```python
from build123d import *

# Parameters (mm, degrees)
EXTRUDE_1_DEPTH              = 5
SKETCH_2_R                   = 1.525
CUT_EXTRUDE_1_DEPTH          = 6
SKETCH_3_R                   = 48.25
EXTRUDE_2_DEPTH              = 5
SKETCH_4_R                   = 32
CUT_EXTRUDE_2_DEPTH          = 6
FILLET_1_R                   = 40
SKETCH_9_R                   = 7.5
CUT_EXTRUDE_7_DEPTH          = 6
SKETCH_15_R                  = 1.525
CUT_EXTRUDE_10_DEPTH         = 6
SKETCH_16_R                  = 1.525
SKETCH_16_R_2                = 3.525
CUT_EXTRUDE_11_DEPTH         = 6
SKETCH_17_R                  = 1.525
SKETCH_17_R_2                = 3.525
SKETCH_17_R_3                = 7.5
CUT_EXTRUDE_12_DEPTH         = 6
SKETCH_10_R                  = 1.775
CUT_EXTRUDE_13_DEPTH         = 6
SKETCH_19_R                  = 1.525
CUT_EXTRUDE_14_DEPTH         = 6
HOLE_WIZARD_M3_2_D           = 3.4
HOLE_WIZARD_M3_2_CSINK_D     = 6.6
HOLE_WIZARD_M3_2_CSINK_ANGLE = 90


with BuildPart() as part:
    # 草图1 → 凸台-拉伸1 (new body)
    with BuildSketch(Plane(origin=(0, 0, 0), x_dir=(1, 0, 0), z_dir=(0, 1, 0))):
        with BuildLine():
            ThreePointArc((-78.875, 0), (-86.526835342, -18.473164658), (-105, -26.125))
            Line((-105, -26.125), (105, -26.125))
            Line((105, -26.125), (105, 26.125))
            Line((105, 26.125), (-105, 26.125))
            ThreePointArc((-105, 26.125), (-86.526835342, 18.473164658), (-78.875, 0))
        make_face()
        with BuildLine():
            ThreePointArc((-105, 26.125), (-131.125, 0), (-105, -26.125))
            Line((-105, -26.125), (-105, 26.125))
        make_face()
        with BuildLine():
            Line((-105, 26.125), (-105, -26.125))
            ThreePointArc((-105, -26.125), (-86.526835342, -18.473164658), (-78.875, 0))
            ThreePointArc((-78.875, 0), (-86.526835342, 18.473164658), (-105, 26.125))
        make_face()
        with BuildLine():
            ThreePointArc((-105, 26.125), (-131.125, 0), (-105, -26.125))
            Line((-105, -26.125), (-105, 26.125))
        make_face()
        with BuildLine():
            Line((-105, 26.125), (-105, -26.125))
            ThreePointArc((-105, -26.125), (-86.526835342, -18.473164658), (-78.875, 0))
            ThreePointArc((-78.875, 0), (-86.526835342, 18.473164658), (-105, 26.125))
        make_face()
    extrude(amount=EXTRUDE_1_DEPTH)

    # 草图2 → 切除-拉伸1 (cut, through all)
    with BuildSketch(Plane(origin=(0, 5, 0), x_dir=(1, 0, 0), z_dir=(0, 1, 0))):
        with Locations((-91.5, 0)):
            Circle(SKETCH_2_R)
        with Locations((-98.25, -11.691342951)):
            Circle(SKETCH_2_R)
        with Locations((-111.75, -11.691342951)):
            Circle(SKETCH_2_R)
        with Locations((-118.5, 0)):
            Circle(SKETCH_2_R)
        with Locations((-111.75, 11.691342951)):
            Circle(SKETCH_2_R)
        with Locations((-98.25, 11.691342951)):
            Circle(SKETCH_2_R)
    extrude(amount=-CUT_EXTRUDE_1_DEPTH, mode=Mode.SUBTRACT)

    # 草图3 → 凸台-拉伸2 (add)
    with BuildSketch(Plane(origin=(0, 5, 0), x_dir=(1, 0, 0), z_dir=(0, 1, 0))):
        with Locations((105, 0)):
            Circle(SKETCH_3_R)
    extrude(amount=-EXTRUDE_2_DEPTH)

    # 草图4 → 切除-拉伸2 (cut, through all)
    with BuildSketch(Plane(origin=(0, 5, 0), x_dir=(1, 0, 0), z_dir=(0, 1, 0))):
        with Locations((105, 0)):
            Circle(SKETCH_4_R)
    extrude(amount=-CUT_EXTRUDE_2_DEPTH, mode=Mode.SUBTRACT)

    # 圆角1
    fillet_1_edges = [part.edges().sort_by_distance(p)[0] for p in [
        (64.43465919, 2.5, 26.125),
        (64.43465919, 2.5, -26.125),
    ]]
    fillet(fillet_1_edges, radius=FILLET_1_R)

    # 草图9 → 切除-拉伸7 (cut, through all)
    with BuildSketch(Plane(origin=(0, 5, 0), x_dir=(1, 0, 0), z_dir=(0, 1, 0))):
        with Locations((-105, 0)):
            Circle(SKETCH_9_R)
    extrude(amount=-CUT_EXTRUDE_7_DEPTH, mode=Mode.SUBTRACT)

    # 草图15 → 切除-拉伸10 (cut, through all)
    with BuildSketch(Plane(origin=(0, 5, 0), x_dir=(1, 0, 0), z_dir=(0, 1, 0))):
        with Locations((-123.619546181, 10.75)):
            Circle(SKETCH_15_R)
        with Locations((-105, 21.5)):
            Circle(SKETCH_15_R)
        with Locations((-86.380453819, 10.75)):
            Circle(SKETCH_15_R)
        with Locations((-86.380453819, -10.75)):
            Circle(SKETCH_15_R)
        with Locations((-105, -21.5)):
            Circle(SKETCH_15_R)
        with Locations((-123.619546181, -10.75)):
            Circle(SKETCH_15_R)
    extrude(amount=-CUT_EXTRUDE_10_DEPTH, mode=Mode.SUBTRACT)

    # 草图16 → 切除-拉伸11 (cut, through all)
    with BuildSketch(Plane(origin=(0, 5, 0), x_dir=(1, 0, 0), z_dir=(0, 1, 0))):
        with Locations((-111.75, 11.691342951)):
            Circle(SKETCH_16_R)
        with Locations((-111.75, 11.691342951)):
            Circle(SKETCH_16_R_2)
        with Locations((-111.75, 11.691342951)):
            Circle(SKETCH_16_R, mode=Mode.SUBTRACT)
        with Locations((-98.25, 11.691342951)):
            Circle(SKETCH_16_R_2)
        with Locations((-98.25, 11.691342951)):
            Circle(SKETCH_16_R, mode=Mode.SUBTRACT)
        with Locations((-98.25, 11.691342951)):
            Circle(SKETCH_16_R)
        with Locations((-91.5, 0)):
            Circle(SKETCH_16_R)
        with Locations((-91.5, 0)):
            Circle(SKETCH_16_R_2)
        with Locations((-91.5, 0)):
            Circle(SKETCH_16_R, mode=Mode.SUBTRACT)
        with Locations((-98.25, -11.691342951)):
            Circle(SKETCH_16_R_2)
        with Locations((-98.25, -11.691342951)):
            Circle(SKETCH_16_R, mode=Mode.SUBTRACT)
        with Locations((-111.75, -11.691342951)):
            Circle(SKETCH_16_R_2)
        with Locations((-111.75, -11.691342951)):
            Circle(SKETCH_16_R, mode=Mode.SUBTRACT)
        with Locations((-111.75, -11.691342951)):
            Circle(SKETCH_16_R)
        with Locations((-118.5, 0)):
            Circle(SKETCH_16_R_2)
        with Locations((-118.5, 0)):
            Circle(SKETCH_16_R, mode=Mode.SUBTRACT)
        with Locations((-118.5, 0)):
            Circle(SKETCH_16_R)
    extrude(amount=-CUT_EXTRUDE_11_DEPTH, mode=Mode.SUBTRACT)

    # 草图17 → 切除-拉伸12 (cut, through all)
    with BuildSketch(Plane(origin=(0, 5, 0), x_dir=(1, 0, 0), z_dir=(0, 1, 0))):
        with BuildLine():
            ThreePointArc((-105, 26.125), (-131.125, 0), (-105, -26.125))
            Line((-105, -26.125), (46.557319748, -26.125))
            ThreePointArc((46.557319748, -26.125), (60.719472559, -28.715998038), (73.046919862, -36.153328612))
            ThreePointArc((73.046919862, -36.153328612), (56.75, 0), (73.046919862, 36.153328612))
            ThreePointArc((73.046919862, 36.153328612), (60.719472559, 28.715998038), (46.557319748, 26.125))
            Line((46.557319748, 26.125), (-105, 26.125))
        make_face()
        with Locations((-105, -21.5)):
            Circle(SKETCH_17_R, mode=Mode.SUBTRACT)
        with Locations((-123.619546181, -10.75)):
            Circle(SKETCH_17_R, mode=Mode.SUBTRACT)
        with Locations((-111.75, -11.691342951)):
            Circle(SKETCH_17_R_2, mode=Mode.SUBTRACT)
        with Locations((-98.25, -11.691342951)):
            Circle(SKETCH_17_R_2, mode=Mode.SUBTRACT)
        with Locations((-118.5, 0)):
            Circle(SKETCH_17_R_2, mode=Mode.SUBTRACT)
        with Locations((-105, 0)):
            Circle(SKETCH_17_R_3, mode=Mode.SUBTRACT)
        with Locations((-86.380453819, -10.75)):
            Circle(SKETCH_17_R, mode=Mode.SUBTRACT)
        with Locations((-123.619546181, 10.75)):
            Circle(SKETCH_17_R, mode=Mode.SUBTRACT)
        with Locations((-111.75, 11.691342951)):
            Circle(SKETCH_17_R_2, mode=Mode.SUBTRACT)
        with Locations((-98.25, 11.691342951)):
            Circle(SKETCH_17_R_2, mode=Mode.SUBTRACT)
        with Locations((-91.5, 0)):
            Circle(SKETCH_17_R_2, mode=Mode.SUBTRACT)
        with Locations((-86.380453819, 10.75)):
            Circle(SKETCH_17_R, mode=Mode.SUBTRACT)
        with Locations((-105, 21.5)):
            Circle(SKETCH_17_R, mode=Mode.SUBTRACT)
    extrude(amount=-CUT_EXTRUDE_12_DEPTH, mode=Mode.SUBTRACT)

    # 草图10 → 切除-拉伸13 (cut, through all)
    with BuildSketch(Plane(origin=(0, 5, 0), x_dir=(1, 0, 0), z_dir=(0, 1, 0))):
        with Locations((73.533748237, 31.466251763)):
            Circle(SKETCH_10_R)
        with Locations((105, 44.5)):
            Circle(SKETCH_10_R)
        with Locations((136.466251763, 31.466251763)):
            Circle(SKETCH_10_R)
        with Locations((136.466251763, -31.466251763)):
            Circle(SKETCH_10_R)
        with Locations((73.533748237, -31.466251763)):
            Circle(SKETCH_10_R)
        with Locations((60.5, 0)):
            Circle(SKETCH_10_R)
        with Locations((149.5, 0)):
            Circle(SKETCH_10_R)
        with Locations((105, -44.5)):
            Circle(SKETCH_10_R)
    extrude(amount=-CUT_EXTRUDE_13_DEPTH, mode=Mode.SUBTRACT)

    # 草图19 → 切除-拉伸14 (cut, through all)
    with BuildSketch(Plane(origin=(0, 5, 0), x_dir=(1, 0, 0), z_dir=(0, 1, 0))):
        with Locations((122.02941274, 41.112639197)):
            Circle(SKETCH_19_R)
        with Locations((146.112639197, 17.02941274)):
            Circle(SKETCH_19_R)
        with Locations((146.112639197, -17.02941274)):
            Circle(SKETCH_19_R)
        with Locations((122.02941274, -41.112639197)):
            Circle(SKETCH_19_R)
        with Locations((87.97058726, -41.112639197)):
            Circle(SKETCH_19_R)
        with Locations((63.887360803, -17.02941274)):
            Circle(SKETCH_19_R)
        with Locations((63.887360803, 17.02941274)):
            Circle(SKETCH_19_R)
        with Locations((87.97058726, 41.112639197)):
            Circle(SKETCH_19_R)
    extrude(amount=-CUT_EXTRUDE_14_DEPTH, mode=Mode.SUBTRACT)

    # M3 开槽沉头木螺钉的锥形沉头孔2 (through all)
    with Locations(Plane(origin=(0, 5, 0), x_dir=(1, 0, 0), z_dir=(0, 1, 0))):
        with Locations((87.97058726, 41.112639197), (122.02941274, 41.112639197), (146.112639197, 17.02941274), (146.112639197, -17.02941274), (122.02941274, -41.112639197), (87.97058726, -41.112639197), (63.887360803, -17.02941274), (63.887360803, 17.02941274)):
            CounterSinkHole(HOLE_WIZARD_M3_2_D / 2, HOLE_WIZARD_M3_2_CSINK_D / 2, counter_sink_angle=HOLE_WIZARD_M3_2_CSINK_ANGLE)


solid = part.part
```
Design review of the part built by this model. Coordinates are the model's own, in mm. Give positions to 0.01 mm unless a question says otherwise; leave off trailing zeros. Write each loop counter-clockwise with the first axis right and the second up, starting at its lowest first coordinate (ties: lowest second). Pieces come first, ordered by that corner, then holes. Notation, with made-up numbers: (85, -16) -> (143, -16) arc R17 ccw to (143, -12) -> close; hole circle Ø2 at (18.25, 60.5). An arc over 180 degrees is marked (long way). Answer in a Markdown table with one row per item.
(1) To check wall thickness, follow probe 1 along X at (y, z) = (3.1, 0) (3 decimals); probe 2 along Z at (x, y) = (105, 2.8) (3 decimals); probe 3 along X at (y, z) = (2.35, 40). State the ranges of each line that lie inside material, in increasing order.
Results:
| item | result |
|---|---|
| probe 1 | 56.75 to 58.725, 62.275 to 73, 137 to 147.725, 151.275 to 153.25 |
| probe 2 | -48.25 to -46.275, -42.725 to -32, 32 to 42.725, 46.275 to 48.25 |
| probe 3 | 78.02 to 86.69, 89.26 to 120.74, 123.31 to 131.98 |
(2) Consider section A-A (z = 0). State the section outline as (x, y) points (3 decimals), then the cut area to 3 significant figures.
Results:
| item | result |
|---|---|
| outline | (56.75, 0) -> (58.725, 0) -> (58.725, 5) -> (56.75, 5) -> close; (62.275, 0) -> (73, 0) -> (73, 5) -> (62.275, 5) -> close; (137, 0) -> (147.725, 0) -> (147.725, 5) -> (137, 5) -> close; (151.275, 0) -> (153.25, 0) -> (153.25, 5) -> (151.275, 5) -> close |
| area | 127 mm2 |
(3) Consider section B-B (x = 110.5). State the section outline as (y, z) points, then the cut area to 3 significant figures.
Results:
| item | result |
|---|---|
| outline | (0, -47.94) -> (5, -47.94) -> (5, -31.52) -> (0, -31.52) -> close; (0, 31.52) -> (5, 31.52) -> (5, 47.94) -> (0, 47.94) -> close |
| area | 164 mm2 |
(4) Clearance check with flat-ended pins moving along their axes: pin 1 (4 mm diameter, centred on x = 146.11, z = -17.03, fed in from -Y); pin 2 (3 mm diameter, centred on y = 4, z = -35.5, fed in from -X); pin 3 (1 mm diameter, centred on y = 1, z = 9, fed in from -X); pin 4 (1 mm diameter, centred on x = 96, y = 3.5, fed in from +Z). State where each tip first meets the part, or that it passes through.
Results:
| item | result |
|---|---|
| pin 1 | y = 0 |
| pin 2 | x = 70.76 |
| pin 3 | x = 57.5 |
| pin 4 | z = 47.5 |
(5) Consider section C-C (z = 10). State the section outline as (x, y) points, then the cut area to 3 significant figures.
Results:
| item | result |
|---|---|
| outline | (57.8, 0) -> (74.6, 0) -> (74.6, 5) -> (57.8, 5) -> close; (135.4, 0) -> (152.2, 0) -> (152.2, 5) -> (135.4, 5) -> close |
| area | 168 mm2 |
(6) Mouldability with a two-part tool opening along X and no side actions: class faces 1 (the cylindrical face through (134.693, 2.535, 31.388)), 2 (the flat face through (115, 5, 31)) as +X half, -X half, draft (parallel to the pull), parting line (faces both ways), or undercut.
Results:
| item | result |
|---|---|
| face 1 | undercut |
| face 2 | draft |
